Geometry check sheet. Reference: the model listing, model coordinates, mm. A direction names the side the tool comes from. Give positions to 0.01 mm unless a question says otherwise; leave off trailing zeros. Write each loop counter-clockwise with the first axis right and the second up, starting at its lowest first coordinate (ties: lowest second). Pieces come first, ordered by that corner, then holes.
(1) Thickness scan on line 1 along Z through (x, y) = (789, 0); line 2 along Z through (x, y) = (574, 0); line 3 along Y through (x, z) = (233.5, -1.5). Record the ranges inside material, lowest first.
(2) Tool access check on faces 1 (the flat face through (812.8, 17, -6)), 2 (the cylindrical face through (778.364, -13.858, -10.626)). Record the directions out of +Z, -Z, +X, -X, +Y, -Y that give a thin tool (end or side, any length) a straight path to the whole face; none if there is none.
(3) Depth check by flat-ended pin: P1, Ø1.5, axis at x = 499, y = -12.5, coming from the +Z side; P2, Ø3, axis at y = -13, z = -5.5, coming from the +X side; P3, Ø8, axis at x = 646.5, y = -3.5, coming from the +Z side; P4, Ø6, axis at x = 268, z = 2, coming from the -Y side. Enter the tip coordinate at first touch or a pass-through.
(4) Mould release check, pull along Y, two halves, no side actions. Record for faces 3 (the cylindrical face through (400.71, -15.12, -11.59)), 4 (the flat face through (0, 10, -11)), 5 (the cylindrical face through (376.676, -14.692, 0.647)): +Y half, -Y half, draft (parallel to the pull), parting line (faces both ways), or undercut.
(5) Cross-section at C-C (x = 608). Record the boundary of the cut face in (y, z), and give its area (3 significant figures).
(6) Cross-section at A-A (y = 0). Record the boundary of the cut face in (x, z).
```python
from build123d import *

# Parameters (mm, degrees)
F0_R     = 19.05
F1_DEPTH = 812.8
F2_R     = 17.4625
F3_DEPTH = 69.85
F4_R     = 14.7066
F5_DEPTH = 742.951


with BuildPart() as f1:
    # F0 (on Right) → F1 (new body)
    with BuildSketch(Plane.YZ):
        Circle(F0_R)
    extrude(amount=F1_DEPTH)

    # F2 (on face) → F3 (cut)
    with BuildSketch(Plane.YZ.offset(812.8)):
        Circle(F2_R)
    extrude(amount=-F3_DEPTH, mode=Mode.SUBTRACT)

    # F4 (on face) → F5 (cut, through all)
    with BuildSketch(Plane.YZ.offset(742.95)):
        Circle(F4_R)
    extrude(amount=-F5_DEPTH, mode=Mode.SUBTRACT)


solid = f1.part
```
Reply:
1. line 1: z = -19.05 to -17.46, 17.46 to 19.05
1. line 2: z = -19.05 to -14.71, 14.71 to 19.05
1. line 3: y = -18.99 to -14.63, 14.63 to 18.99
2. face 1: +Z, -Z, +X, +Y, -Y
2. face 2: +X
3. P1: stops at z = 14.99
3. P2: stops at x = 742.95
3. P3: stops at z = 19.05
3. P4: stops at y = -19.05
4. face 3: parting line
4. face 4: draft
4. face 5: undercut
5. outline: circle Ø38.1 at (0, 0); hole circle Ø29.41 at (0, 0)
5. area: 461 mm2
6. outline: (0, -19.05) - (812.8, -19.05) - (812.8, -17.46) - (742.95, -17.46) - (742.95, -14.71) - (0, -14.71) - close; (0, 14.71) - (742.95, 14.71) - (742.95, 17.46) - (812.8, 17.46) - (812.8, 19.05) - (0, 19.05) - close
